Check sheet for the modelled part. Datum: model origin and axes. Units: mm. Give positions to 0.01 mm unless a question says otherwise; leave off trailing zeros. Loops run counter-clockwise (first coordinate to the right, second up) from the corner with the lowest first, then second, coordinate; pieces in that order, holes last. Notation, with made-up numbers: (-9.5, -10) - (-2.5, -10) arc R16 ccw to (-2.5, 12) - close; hole circle Ø8 at (88.5, -37.5). An arc over 180 degrees is marked (long way). Use CSV: the item, a comma, the result in double quotes.
from build123d import *

# Parameters (mm, degrees)
SKETCH1_W           = 48
SKETCH1_H           = 48
SKETCH1_R           = 1.5
SKETCH1_R_2         = 2
BOSS_EXTRUDE1_DEPTH = 3
FILLET1_R           = 10
FILLET2_R           = 10
FILLET3_R           = 10
FILLET4_R           = 10


with BuildPart() as part:
    # Sketch1 → Boss-Extrude1 (new body)
    with BuildSketch(Plane.XY):
        Rectangle(SKETCH1_W, SKETCH1_H)
        with Locations((10, 10)):
            Circle(SKETCH1_R, mode=Mode.SUBTRACT)
        with Locations((-10, 10)):
            Circle(SKETCH1_R, mode=Mode.SUBTRACT)
        with Locations((-10, -10)):
            Circle(SKETCH1_R, mode=Mode.SUBTRACT)
        with Locations((10, -10)):
            Circle(SKETCH1_R, mode=Mode.SUBTRACT)
        with Locations((-16, 16)):
            Circle(SKETCH1_R_2, mode=Mode.SUBTRACT)
        with Locations((16, 16)):
            Circle(SKETCH1_R_2, mode=Mode.SUBTRACT)
        with Locations((16, -16)):
            Circle(SKETCH1_R_2, mode=Mode.SUBTRACT)
        with Locations((-15.708422677, -16)):
            Circle(SKETCH1_R_2, mode=Mode.SUBTRACT)
    extrude(amount=BOSS_EXTRUDE1_DEPTH)

    # Fillet1
    fillet1_edges = [part.edges().sort_by_distance(p)[0] for p in [
        (-24, 24, 1.5),
    ]]
    fillet(fillet1_edges, radius=FILLET1_R)

    # Fillet2
    fillet2_edges = [part.edges().sort_by_distance(p)[0] for p in [
        (24, 24, 1.5),
    ]]
    fillet(fillet2_edges, radius=FILLET2_R)

    # Fillet3
    fillet3_edges = [part.edges().sort_by_distance(p)[0] for p in [
        (24, -24, 1.5),
    ]]
    fillet(fillet3_edges, radius=FILLET3_R)

    # Fillet4
    fillet4_edges = [part.edges().sort_by_distance(p)[0] for p in [
        (-24, -24, 1.5),
    ]]
    fillet(fillet4_edges, radius=FILLET4_R)


solid = part.part
1. Sectioned sample at B-B, the plane z = 0.5. State how many separate pieces and enclosed holes the cut face has, and give its area (3 significant figures).
Completed:
separate pieces,"1"
enclosed holes,"8"
area,"2,140 mm²"
2. Scan lines: line 1 along Y through (x, z) = (10, 0.85); line 2 along X through (y, z) = (-9, 0.95); line 3 along Y through (x, z) = (-14.5, 0.5). Record each from-to range of solid material in increasing order.
Completed:
line 1,"y = -24 to -11.5, -8.5 to 8.5, 11.5 to 24"
line 2,"x = -24 to -11.12, -8.88 to 8.88, 11.12 to 24"
line 3,"y = -23.99 to -17.59, -14.41 to 14.68, 17.32 to 23.99"
3. Release check for a two-part mould opening along Y. For faces 1 (the face through (20.99, 21.15, 1.52)), 2 (the face through (21.15, -20.99, 1.52)), 3 (the face through (0, 0, 0)), 4 (the face through (8.8, 9.1, 1.5)) record: released by +Y, released by -Y, zero draft, split by the parting line, or undercut.
Completed:
face 1,"released by +Y"
face 2,"released by -Y"
face 3,"zero draft"
face 4,"undercut"
4. Go/stop test with flat-tipped pins: pin 1 Ø2.5 at (x, y) = (-16, 16) entering from +Z; pin 2 Ø1.5 at (x, z) = (-19, 2) entering from -Y. Record where each tip stops, or that it passes through.
Completed:
pin 1,"passes through"
pin 2,"stops at y = -23.05"
5. Sectioned sample at A-A, the plane y = -10. Record the boundary of the cut face in (x, z), and give its area (3 significant figures).
Completed:
outline,"(-24, 0) - (-11.5, 0) - (-11.5, 3) - (-24, 3) - close; (-8.5, 0) - (8.5, 0) - (8.5, 3) - (-8.5, 3) - close; (11.5, 0) - (24, 0) - (24, 3) - (11.5, 3) - close"
area,"126 mm²"
6. Sectioned sample at D-D, the plane y = 20.5. Record the boundary of the cut face in (x, z), and give its area (3 significant figures).
Completed:
outline,"(-21.6, 0) - (21.6, 0) - (21.6, 3) - (-21.6, 3) - close"
area,"130 mm²"
